```python
from build123d import *

# Parameters (mm, degrees)
EXTRUDE_1_DEPTH = 5
SKETCH_19_W     = 5
SKETCH_19_H     = 18
EXTRUDE_2_DEPTH = 1.5
FILLET_2_R      = 2


with BuildPart() as part:
    # 扫描2: sweep along a path in 草图1
    with BuildLine(Plane.XY) as sweep_2_path:
        Line((11.886241035, 20.255064977), (10.916442642, 25.755064977))
        ThreePointArc((10.916442642, 25.755064977), (5.020643415, 30.27907084), (0, 24.8))
        Line((0, 24.8), (0, 0))
        Line((0, 0), (0, -3))
    # 草图13 → 扫描2 (sweep)
    with BuildSketch(Plane(origin=(0, -3, 0), x_dir=(1, 0, 0), z_dir=(0, 1, 0))):
        with BuildLine():
            Line((-1, -2.5), (1, -2.5))
            ThreePointArc((1, -2.5), (2.5, 0), (1, 2.5))
            Line((1, 2.5), (-1, 2.5))
            ThreePointArc((-1, 2.5), (-2.5, 0), (-1, -2.5))
        make_face()
    sweep(path=sweep_2_path.line)

    # 扫描4: sweep along a path in 草图15
    with BuildLine(Plane.XY) as sweep_4_path:
        Line((0, 0), (11, 0))
    # 草图16 → 扫描4 (sweep)
    with BuildSketch(Plane(origin=(11, 0, 0), x_dir=(0, 0, -1), z_dir=(1, 0, 0))):
        with BuildLine():
            Line((-2.5, -1), (-2.5, 1))
            ThreePointArc((-2.5, 1), (0, 2.5), (2.5, 1))
            Line((2.5, 1), (2.5, -1))
            ThreePointArc((2.5, -1), (0, -2.5), (-2.5, -1))
        make_face()
    sweep(path=sweep_4_path.line)

    # 草图17 → 凸台-拉伸1 (add)
    with BuildSketch(Plane(origin=(11, 0, 0), x_dir=(0, 0, -1), z_dir=(1, 0, 0))):
        with BuildLine():
            Line((-2.5, 1.555522876), (-2.5, -1.555522876))
            ThreePointArc((-2.5, -1.555522876), (0, -2.8), (2.5, -1.555522876))
            Line((2.5, -1.555522876), (2.5, 1.555522876))
            ThreePointArc((2.5, 1.555522876), (0, 2.8), (-2.5, 1.555522876))
        make_face()
    extrude(amount=-EXTRUDE_1_DEPTH)

    # 草图19 → 凸台-拉伸2 (add)
    with BuildSketch(Plane(origin=(1, 0, 0), x_dir=(0, 0, -1), z_dir=(1, 0, 0))):
        with Locations((0, 14)):
            Rectangle(SKETCH_19_W, SKETCH_19_H)
    extrude(amount=EXTRUDE_2_DEPTH)

    # 圆角2
    # the kernel refuses this fillet: 2 mm, written as the material it takes off along each edge
    with BuildSketch(Plane(origin=(17.795087554, 21.296954043, 2.5), x_dir=(0, 0, -1), z_dir=(-0.9848077530122092, -0.17364817766692373, 0))) as fillet_2_piece_1:
        with BuildLine():
            CenterArc((FILLET_2_R, -FILLET_2_R), FILLET_2_R, 90, 90)
            Line((0, -FILLET_2_R), (0, 0))
            Line((0, 0), (FILLET_2_R, 0))
        make_face()
    extrude(amount=12, mode=Mode.SUBTRACT)
    with BuildSketch(Plane(origin=(12.214510286, 20.312947703, 0), x_dir=(0.9423506208781959, 0.16616183974819204, -0.29045748456869663), z_dir=(0.2860447827236766, 0.05043741288507259, 0.9568878981667733))) as fillet_2_piece_2:
        with BuildLine():
            CenterArc((2.833333333 - FILLET_2_R, FILLET_2_R), FILLET_2_R, 270, 90)
            Line((2.833333333 - FILLET_2_R, 0), (2.833333333, 0))
            Line((2.833333333, 0), (2.833333333, FILLET_2_R))
        make_face()
    revolve(axis=Axis((12.214510286, 20.312947703, 0), (-0.173648177666923, 0.9848077530122094, 0)), revolution_arc=326.229306127, mode=Mode.SUBTRACT)
    with BuildSketch(Plane(origin=(5.977394517, 19.213175911, -2.5), x_dir=(-0.17364817766692373, 0.9848077530122092, 0), z_dir=(0.9848077530122092, 0.17364817766692373, 0))) as fillet_2_piece_3:
        with BuildLine():
            CenterArc((FILLET_2_R, FILLET_2_R), FILLET_2_R, 180, 90)
            Line((0, FILLET_2_R), (0, 0))
            Line((0, 0), (FILLET_2_R, 0))
        make_face()
    extrude(amount=12, mode=Mode.SUBTRACT)
    with BuildSketch(Plane(origin=(11, -6.555522876, 2.5), x_dir=(0, 0, -1), z_dir=(0, 1, 0))) as fillet_2_piece_4:
        with BuildLine():
            CenterArc((FILLET_2_R, FILLET_2_R), FILLET_2_R, 180, 90)
            Line((0, FILLET_2_R), (0, 0))
            Line((0, 0), (FILLET_2_R, 0))
        make_face()
    extrude(amount=13.111045751, mode=Mode.SUBTRACT)
    with BuildSketch(Plane(origin=(11, 6.555522876, -2.5), x_dir=(-1, 0, 0), z_dir=(0, -1, 0))) as fillet_2_piece_5:
        with BuildLine():
            CenterArc((FILLET_2_R, -FILLET_2_R), FILLET_2_R, 90, 90)
            Line((0, -FILLET_2_R), (0, 0))
            Line((0, 0), (FILLET_2_R, 0))
        make_face()
    extrude(amount=13.111045751, mode=Mode.SUBTRACT)
    with BuildSketch(Plane(origin=(11, -0.333333333, 0), x_dir=(0, -0.8131785022115455, -0.582014367125922), z_dir=(0, -0.582014367125922, 0.8131785022115455))) as fillet_2_piece_6:
        with BuildLine():
            CenterArc((3.133333333 - FILLET_2_R, -FILLET_2_R), FILLET_2_R, 0, 90)
            Line((3.133333333, -FILLET_2_R), (3.133333333, 0))
            Line((3.133333333, 0), (3.133333333 - FILLET_2_R, 0))
        make_face()
    revolve(axis=Axis((11, -0.333333333, 0), (1, 0, 0)), revolution_arc=288.815304863, mode=Mode.SUBTRACT)
    with BuildSketch(Plane(origin=(11, 0.333333333, 0), x_dir=(0, 0.8131785022115376, 0.5820143671259329), z_dir=(0, 0.5820143671259329, -0.8131785022115376))) as fillet_2_piece_7:
        with BuildLine():
            CenterArc((3.133333333 - FILLET_2_R, -FILLET_2_R), FILLET_2_R, 0, 90)
            Line((3.133333333 - FILLET_2_R, 0), (3.133333333, 0))
            Line((3.133333333, 0), (3.133333333, -FILLET_2_R))
        make_face()
    revolve(axis=Axis((11, 0.333333333, 0), (1, 0, 0)), revolution_arc=288.815304863, mode=Mode.SUBTRACT)
    with BuildSketch(Plane(origin=(11.557971784, 20.197182251, 0), x_dir=(-0.9423506208781961, -0.16616183974819207, 0.2904574845686964), z_dir=(-0.2860447827236764, -0.05043741288507257, -0.9568878981667737))) as fillet_2_piece_8:
        with BuildLine():
            CenterArc((2.833333333 - FILLET_2_R, FILLET_2_R), FILLET_2_R, 270, 90)
            Line((2.833333333, FILLET_2_R), (2.833333333, 0))
            Line((2.833333333, 0), (2.833333333 - FILLET_2_R, 0))
        make_face()
    revolve(axis=Axis((11.557971784, 20.197182251, 0), (-0.17364817766692306, 0.9848077530122095, 0)), revolution_arc=326.229306127, mode=Mode.SUBTRACT)


solid = part.part
```
Can you work these out from the model? Positions are in its coordinate system, mm. A direction names the side the tool comes from. Coordinates: 2 decimals unless noted, no trailing zeros. Loops run counter-clockwise (first coordinate to the right, second up) from the corner with the lowest first, then second, coordinate; pieces in that order, holes last. Notation, with made-up numbers: (60, 80) -> (91, 80) arc R24 ccw to (91, 95) -> close; hole circle Ø6 at (35.5, 87). An arc over 180 degrees is marked (long way). Put each result on its own line as item: value. Start each with the question number.
Q1. For faces 1 (the face through (8.76, 23.58, -0.04)), 2 (the face through (2.5, -2.7, 0)), 3 (the face through (10.13, 0.02, -2.15)), which set-ups out of +Z, -Z, +X, -X, +Y, -Y let a thin tool reach every point of the face, with its end or its side?
Q2. If I drill on line 1 (X direction, y = 24, z = 1); line 2 (X direction, y = 27, z = -1.8); line 3 (Y direction, x = 3.25, z = 1), over which ranges is the centre line in solid material (lowest first)? Write a range as [from, to].
Q3. I'm going to push flat-ended pins straight in: P1, Ø1.7, axis at x = 1.5, z = -1, coming from the +Y side; P2, Ø2.5, axis at y = 10.5, z = -1, coming from the +X side; P3, Ø0.9, axis at y = -1.5, z = 0.5, coming from the -X side; P4, Ø1.5, axis at x = 7, z = 1, coming from the +Y side. Where does each tip first touch, or does it pass through?
Q4. Thinking about a two-plate mould opening in Y: for faces 4 (the face through (2, 5, -2)), 5 (the face through (4.1, -2.5, 0)), 6 (the face through (2, 15, -2.5)), which applies, pulls with the +Y half, pulls with the -Y half, needs draft (parallel to the pull), parting line crosses it, or undercut?
Q5. I want a section at A-A (y = 6). Write out the boundary of the cut face in (x, z).
Taken from the geometry:
1. face 1: none
1. face 2: -Y
1. face 3: -Z, +X, -Y
2. line 1: x = [-2.32, 2.32], [8.87, 13.58]
2. line 2: x = [-1.52, 2.59], [8.41, 12.52]
2. line 3: y = [-2.32, 2.32], [27.05, 32.29]
3. P1: stops at y = 32.04
3. P2: stops at x = 2.5
3. P3: stops at x = -2.5
3. P4: stops at y = 32.7
4. face 4: undercut
4. face 5: pulls with the -Y half
4. face 6: needs draft
5. outline: (-1, -2.5) -> (2.5, -2.5) -> (2.5, 2.5) -> (-1, 2.5) arc R2.83 ccw to start
